Part model, mm, in its own coordinate system. Face numbers are marked on the shaded views. A direction names the side the tool comes from. Give positions to 0.01 mm unless a question says otherwise; leave off trailing zeros. Order: outer loops, then holes, each group sorted by start corner. A loop starts at its lowest first (then second) coordinate and runs counter-clockwise, first axis right, second up.
from build123d import *

# Parameters (mm, degrees)
BOSS_EXTRUDE1_DEPTH = 8
SKETCH4_W           = 32
SKETCH4_H           = 12
BOSS_EXTRUDE3_DEPTH = 9
RIB1_START          = -4
RIB1_DEPTH          = 8
FILLET1_R           = 12
SKETCH8_R           = 6
CUT_EXTRUDE1_DEPTH  = 9


# Read off the part's stored shape, not the designer's step: Rib1
with BuildPart() as part:
    # Sketch1 → Boss-Extrude1 (new body)
    with BuildSketch(Plane.XY):
        Polygon((-55, 22.5), (55, 22.5), (55, -22.5), (4, -48.5), (-4, -48.5), (-55, -22.5), align=None)
    extrude(amount=-BOSS_EXTRUDE1_DEPTH)

    # Sketch2 → Loft1 section 0
    with BuildSketch(Plane.XY):
        with BuildLine():
            Line((-46, -15.311496361), (46, -15.311496361))
            Line((46, -15.311496361), (46, -23.311496361))
            Line((46, -23.311496361), (-46, -23.311496361))
            Line((-46, -23.311496361), (-46, -15.311496361))
        make_face()
    # Sketch3 → Loft1 section 1
    with BuildSketch(Plane.XY.offset(36)):
        with BuildLine():
            Line((-4, -15.311496361), (4, -15.311496361))
            Line((4, -15.311496361), (4, -23.311496361))
            Line((4, -23.311496361), (-4, -23.311496361))
            Line((-4, -23.311496361), (-4, -15.311496361))
        make_face()
    loft()

    # Sketch4 → Boss-Extrude3 (add)
    with BuildSketch(Plane.XY.offset(36)):
        with Locations((0, -17.311496361)):
            Rectangle(SKETCH4_W, SKETCH4_H)
    extrude(amount=BOSS_EXTRUDE3_DEPTH)

    # Sketch6 → Loft3 section 0
    with BuildSketch(Plane.XY):
        with BuildLine():
            Line((-4, -23.311496361), (4, -23.311496361))
            Line((4, -23.311496361), (4, -48.5))
            Line((4, -48.5), (-4, -48.5))
            Line((-4, -48.5), (-4, -23.311496361))
        make_face()
    # Sketch5 → Loft3 section 1
    with BuildSketch(Plane.XY.offset(45)):
        with BuildLine():
            Line((-4, -35.311496361), (4, -35.311496361))
            Line((4, -35.311496361), (4, -23.311496361))
            Line((4, -23.311496361), (-4, -23.311496361))
            Line((-4, -23.311496361), (-4, -35.311496361))
        make_face()
    loft()

    # Rib1 outline → Rib1 (add)
    with BuildSketch(Plane(origin=(0, 0, 0), x_dir=(0, 0, -1), z_dir=(1, 0, 0)).offset(RIB1_START)):
        with BuildLine():
            Line((-30, -11.311496361), (-36, -11.311496361))
            Line((-36, -11.311496361), (-36, -15.311496361))
            Line((-36, -15.311496361), (0, -15.311496361))
            Line((0, -15.311496361), (0, 18.688503639))
            ThreePointArc((0, 18.688503639), (-8.786796565, -2.524699797), (-30, -11.311496361))
        make_face()
    extrude(amount=RIB1_DEPTH)

    # Fillet1
    fillet1_edges = [part.edges().sort_by_distance(p)[0] for p in [
        (-55, 22.5, -4),
        (55, 22.5, -4),
    ]]
    fillet(fillet1_edges, radius=FILLET1_R)

    # Sketch8 → Cut-Extrude1 (cut)
    with BuildSketch(Plane.XY):
        with Locations((-33, 6.5)):
            Circle(SKETCH8_R)
        with Locations((33, 6.5)):
            Circle(SKETCH8_R)
    extrude(amount=-CUT_EXTRUDE1_DEPTH, mode=Mode.SUBTRACT)


solid = part.part
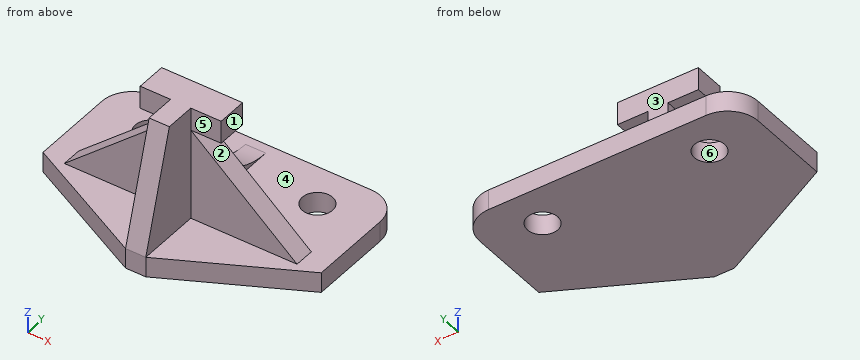
Item 1: Pull direction Y, two halves, no side cores. Call the marked faces 4, 5 and 6: released by +Y, released by -Y, zero draft, split by the parting line, or undercut.
Item 2: Band-saw the part on C-C on y = -8. List the corners of the cut face in (x, z), plus the area to 3 significant figures.
Item 3: Band-saw the part on A-A on z = -2. List the corners of the cut face in (x, y).
Item 4: Which spindle directions (+Z, -Z, +X, -X, +Y, -Y) get a long thin tool onto all of the face, cutting with end or side? Do the marked faces 1, 2 and 3. Say none if no direction does.
Item 5: Band-saw the part on B-B on y = 6.5. List the corners of the cut face in (x, z), plus the area to 3 significant figures.
Item 6: Drop flat-ended pins along their axis: P1, Ø4, axis at y = -17.5, z = 30, coming from the +X side; P2, Ø7, axis at x = 33, y = 6.5, coming from the +Z side; P3, Ø4.5, axis at x = 12, z = 42, coming from the -Y side; P4, Ø8, axis at x = 31, y = -13, coming from the +Z side. Give the stop position or say it passes through.
Item 7: Drill centre lines: probe 1 along X at (y, z) = (6, -3); probe 2 along Z at (x, y) = (-19.5, 2.5); probe 3 along X at (y, z) = (-29.5, 27). Where is each one in solid material? Low to high.
Working result:
1. face 4: zero draft
1. face 5: released by -Y
1. face 6: undercut
2. outline: (-55, -8) - (55, -8) - (55, 0) - (4, 0) - (4, 16.3) - (-4, 16.3) - (-4, 0) - (-55, 0) - close
2. area: 1,010 mm2
3. outline: (-55, -22.5) - (-4, -48.5) - (4, -48.5) - (55, -22.5) - (55, 10.5) arc R12 ccw to (43, 22.5) - (-43, 22.5) arc R12 ccw to (-55, 10.5) - close; hole circle Ø12 at (-33, 6.5); hole circle Ø12 at (33, 6.5)
4. face 1: +Z, +X, +Y, -Y
4. face 2: +X, +Y, -Y
4. face 3: +Z, +X, -X, +Y
5. outline: (-55, -8) - (-39, -8) - (-39, 0) - (-55, 0) - close; (-27, -8) - (27, -8) - (27, 0) - (4, 0) - (4, 2.59) - (-4, 2.59) - (-4, 0) - (-27, 0) - close; (39, -8) - (55, -8) - (55, 0) - (39, 0) - close
5. area: 709 mm2
6. P1: stops at x = 13.33
6. P2: passes through
6. P3: stops at y = -23.31
6. P4: stops at z = 15.66
7. probe 1: x = -55 to -38.98, -27.02 to 27.02, 38.98 to 55
7. probe 2: z = -8 to 0
7. probe 3: x = -4 to 4
